For this review, use the dimensioned drawing (mm, ordinates from the lowest corner) and the shaded views. A direction names the side the tool comes from. Round coordinates to 2 decimals unless told otherwise and drop trailing zeros. Write each loop counter-clockwise with the first axis right and the second up, starting at its lowest first coordinate (ties: lowest second). Pieces come first, ordered by that corner, then holes. Notation, with made-up numbers: (81.5, 18.5) -> (114.5, 18.5) arc R27 cw to (114.5, 53.5) -> close; hole circle Ø4 at (84, 44.5). An arc over 180 degrees is marked (long way). Answer as CSV lines item,"result". Start each with the question number.
Item 1: Wall thickness on probe 1 along X at (y, z) = (26.5, 12.5); probe 2 along Z at (x, y) = (37.9, 20): over which ranges is each line inside the solid? List them lowest first. Write a range as from..to.
Item 2: Take a section at C-C on x = 16.5. Give the boundary of the cut face in (y, z), then the cut area to 3 significant figures.
Item 3: Take a section at A-A on y = 20. Give the boundary of the cut face in (x, z), then the cut area to 3 significant figures.
Item 4: Machinability: for the marked faces 4 and 5, which of the approach directions +Z, -Z, +X, -X, +Y, -Y give a long, thin tool a straight path to every point of the face, cutting with its end or side? Answer none if there is none.
Item 5: Take a section at B-B on z = 10. Give the boundary of the cut face in (x, y).
Item 6: For pin 1 Ø11 at (y, z) = (20, 10) entering from +X, flat-tipped, find the tip position at first contact; note if it passes through.
Item 7: Take a section at D-D on z = 22. Give the boundary of the cut face in (x, y).
Item 8: Mouldability with a two-part tool opening along Y and no side actions: class the marked faces 1, 2 and 3 as +Y half, -Y half, draft (parallel to the pull), parting line (faces both ways), or undercut.
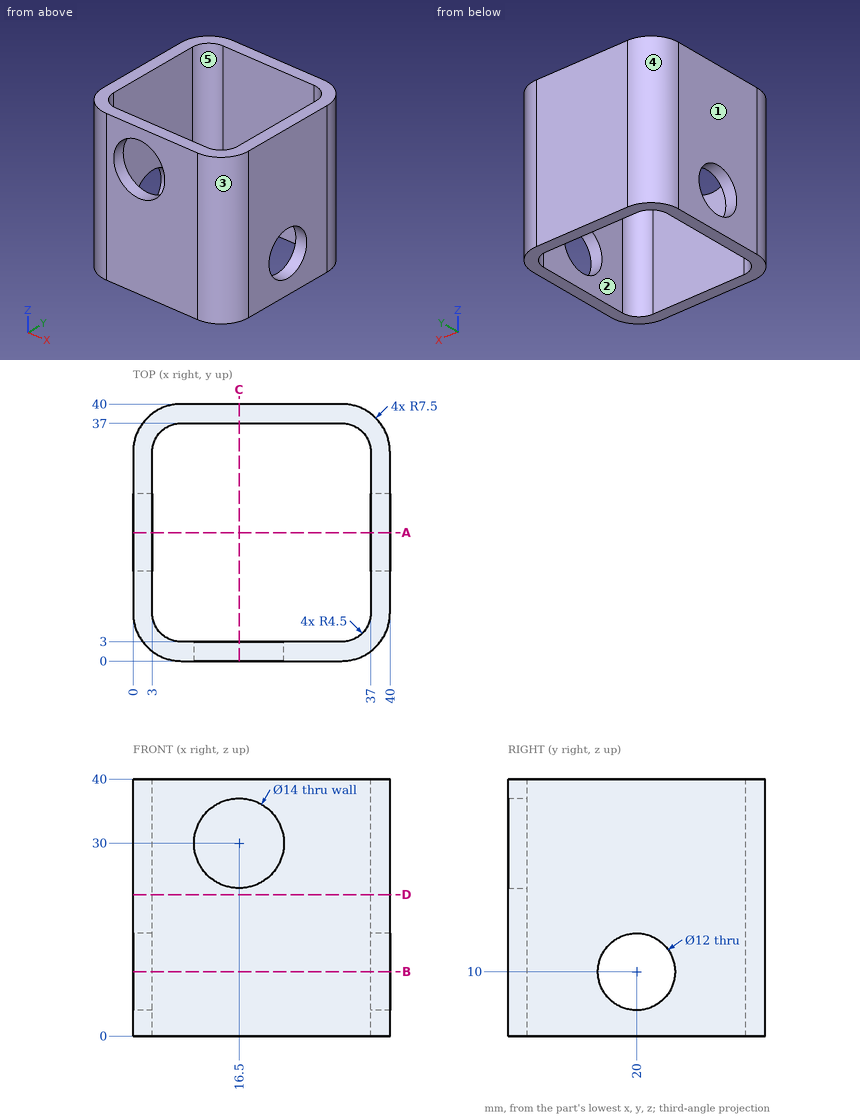
Output values:
1,probe 1,"x = 0..3, 37..40"
1,probe 2,"z = 0..4, 16..40"
2,outline,"(0, 0) -> (3, 0) -> (3, 23) -> (0, 23) -> close; (0, 37) -> (3, 37) -> (3, 40) -> (0, 40) -> close; (37, 0) -> (40, 0) -> (40, 40) -> (37, 40) -> close"
2,area,"198 mm^2"
3,outline,"(0, 0) -> (3, 0) -> (3, 4) -> (0, 4) -> close; (0, 16) -> (3, 16) -> (3, 40) -> (0, 40) -> close; (37, 0) -> (40, 0) -> (40, 4) -> (37, 4) -> close; (37, 16) -> (40, 16) -> (40, 40) -> (37, 40) -> close"
3,area,"168 mm^2"
4,face 4,"+Z, -Z, -X, +Y"
4,face 5,"+Z, -Z"
5,outline,"(0, 7.5) arc R7.5 ccw to (7.5, 0) -> (32.5, 0) arc R7.5 ccw to (40, 7.5) -> (40, 14) -> (37, 14) -> (37, 7.5) arc R4.5 cw to (32.5, 3) -> (7.5, 3) arc R4.5 cw to (3, 7.5) -> (3, 14) -> (0, 14) -> close; (0, 26) -> (3, 26) -> (3, 32.5) arc R4.5 cw to (7.5, 37) -> (32.5, 37) arc R4.5 cw to (37, 32.5) -> (37, 26) -> (40, 26) -> (40, 32.5) arc R7.5 ccw to (32.5, 40) -> (7.5, 40) arc R7.5 ccw to (0, 32.5) -> close"
6,pin 1,"passes through"
7,outline,"(0, 7.5) arc R7.5 ccw to (7.5, 0) -> (32.5, 0) arc R7.5 ccw to (40, 7.5) -> (40, 32.5) arc R7.5 ccw to (32.5, 40) -> (7.5, 40) arc R7.5 ccw to (0, 32.5) -> close; hole (3, 7.5) arc R4.5 ccw to (7.5, 3) -> (32.5, 3) arc R4.5 ccw to (37, 7.5) -> (37, 32.5) arc R4.5 ccw to (32.5, 37) -> (7.5, 37) arc R4.5 ccw to (3, 32.5) -> close"
8,face 1,"draft"
8,face 2,"undercut"
8,face 3,"-Y half"
